Read the model definition and answer for the solid it produces. Units are mm, in the model's axes. A direction names the side the tool comes from. Round coordinates to 2 decimals unless told otherwise and drop trailing zeros. Loops run counter-clockwise (first coordinate to the right, second up) from the corner with the lowest first, then second, coordinate; pieces in that order, holes last. Notation, with made-up numbers: (41, 59) - (65, 59) arc R17 cw to (65, 80) - close; hole circle Ø9 at (-28, -0.75). An arc over 180 degrees is marked (long way). Use CSV: the item, a comma, the result in double quotes. Start each with the question number.
1. Determine the mould class of faces 4 (the flat face through (0, 1, 3.6)), 5 (the cylindrical face through (-3.67, -8.05, -0.02)), 6 (the conical face through (-3.412, 8.373, 2.942)), 7 (the flat face through (-3, 4.5, 0)) for opening direction Y: +Y half, -Y half, draft (parallel to the pull), parting line (faces both ways), or undercut.
2. Given pin 1 Ø1.2 at (x, z) = (2, -0.5) entering from +Y; pin 2 Ø1.7 at (x, z) = (-1.5, -0.5) entering from +Y; pin 3 Ø1.5 at (y, z) = (-3, 2.5) entering from +X, each flat-ended and moving along its own axis, determine where each tip first touches the part or whether it passes through.
3. Find section B-B (z = 0). State how many separate pieces and enclosed holes the cut face has, and give its area (3 significant figures).
4. Consider line 1 along Z through (x, y) = (1.25, -5.5); line 2 along X through (y, z) = (-6, 1); line 3 along X through (y, z) = (5.75, 2). Determine where each line is inside the solid, lowest interval first.
5. A tool of negligible diameter and unlimited length cuts with its end or side. For faces 1 (the flat face through (0, -1, -2.25)), 2 (the flat face through (-3, -4.5, 0)), 3 (the flat face through (-2.75, -5, 0)), from which of +Z, -Z, +X, -X, +Y, -Y can it reach the whole face along a straight path? Write none if from no direction.
6. Find section A-A (y = -0.5). Give the vertices of the cut face in (x, z), and give its area (3 significant figures).
7. Find section C-C (x = 0). Give the vertices of the cut face in (y, z) (3 decimals), and give its area (3 significant figures).
8. Find section D-D (y = 7.25). Give the vertices of the cut face in (x, z), and give its area (3 significant figures).
from build123d import *

# Parameters (mm, degrees)
SKETCH1_W                 = 8.2
SKETCH1_H                 = 7.2
BOSS_EXTRUDE1_DEPTH       = 8.5
SKETCH2_W                 = 0.25
SKETCH2_H                 = 0.25
SKETCH2_H_2               = 4
SKETCH2_W_2               = 5
CHAIN_DEPTH               = 15
F_2_5_MM_DOWEL_DEPTH      = 11.100495037
F_2_5_MM_DOWEL_DEPTH_BACK = 11.100495037
SKETCH3_R                 = 1.25
SKETCH4_R                 = 0.9
STEEL_CABLE_CHANNEL_DEPTH = 11.100495037
CRIMP_WINDOW_DEPTH        = 11.100495037
CRIMP_WINDOW_DEPTH_BACK   = 11.100495037
SKETCH7_W                 = 4.5
SKETCH7_H                 = 9
FILLET6_R                 = 0.75
FILLET7_R                 = 0.5
FILLET9_R                 = 0.5
FILLET3_R                 = 2
FILLET5_R                 = 1.5
CHAMFER1_SIZE             = 0.25
BOSS_EXTRUDE2_START       = 0.005
SKETCH5_R                 = 1.9
SKETCH5_R_2               = 0.9
BOSS_EXTRUDE2_DEPTH       = 0.005


with BuildPart() as part:
    # Sketch1 → Boss-Extrude1 (new, symmetric)
    with BuildSketch(Plane(origin=(0, 0, 0), x_dir=(1, 0, 0), z_dir=(0, 1, 0))):
        Rectangle(SKETCH1_W, SKETCH1_H)
    extrude(amount=BOSS_EXTRUDE1_DEPTH, both=True)

    # Sketch2 → chain (cut)
    with BuildSketch(Plane(origin=(0, 8.5, 0), x_dir=(1, 0, 0), z_dir=(0, 1, 0))):
        with Locations((-2.625, 2.125)):
            Rectangle(SKETCH2_W, SKETCH2_H)
        with Locations((-2.625, 0)):
            Rectangle(SKETCH2_W, SKETCH2_H_2)
        with Locations((0, 2.125)):
            Rectangle(SKETCH2_W_2, SKETCH2_H)
        Rectangle(SKETCH2_W_2, SKETCH2_H_2)
        with Locations((2.625, 2.125)):
            Rectangle(SKETCH2_W, SKETCH2_H)
        with Locations((2.625, 0)):
            Rectangle(SKETCH2_W, SKETCH2_H_2)
        with Locations((2.625, -2.125)):
            Rectangle(SKETCH2_W, SKETCH2_H)
        with Locations((0, -2.125)):
            Rectangle(SKETCH2_W_2, SKETCH2_H)
        with Locations((-2.625, -2.125)):
            Rectangle(SKETCH2_W, SKETCH2_H)
    extrude(amount=-CHAIN_DEPTH, mode=Mode.SUBTRACT)

    # Sketch3 → 2.5 mm dowel (cut, two sides: drawn at the far end of the back side and taken through both)
    with BuildSketch(Plane.XY.offset(-F_2_5_MM_DOWEL_DEPTH_BACK)):
        with Locations((0, 5)):
            Circle(SKETCH3_R)
    extrude(amount=F_2_5_MM_DOWEL_DEPTH + F_2_5_MM_DOWEL_DEPTH_BACK, mode=Mode.SUBTRACT)

    # Sketch4 → steel cable channel (cut, through all)
    with BuildSketch(Plane(origin=(0, 0, 0), x_dir=(1, 0, 0), z_dir=(0, 1, 0))):
        with Locations(Location((0, 0, 0), (0, 0, 270))):
            Circle(SKETCH4_R)
    extrude(amount=-STEEL_CABLE_CHANNEL_DEPTH, mode=Mode.SUBTRACT)

    # Sketch7 → crimp window (cut, two sides: drawn at the far end of the back side and taken through both)
    with BuildSketch(Plane.ZY.offset(-CRIMP_WINDOW_DEPTH_BACK)):
        Rectangle(SKETCH7_W, SKETCH7_H)
    extrude(amount=CRIMP_WINDOW_DEPTH + CRIMP_WINDOW_DEPTH_BACK, mode=Mode.SUBTRACT)

    # Fillet6
    fillet6_edges = [part.edges().sort_by_distance(p)[0] for p in [
        (-2.75, -5.5, -2.25),
        (2.75, -5.5, -2.25),
        (2.75, -5.5, 2.25),
        (-2.75, -5.5, 2.25),
        (-2.75, 6.5, -2.25),
        (-2.75, 6.5, 2.25),
        (2.75, 6.5, 2.25),
        (2.75, 6.5, -2.25),
    ]]
    fillet(fillet6_edges, radius=FILLET6_R)

    # Fillet7
    fillet7_edges = [part.edges().sort_by_distance(p)[0] for p in [
        (2.75, -6.5, 0),
        (2.530330086, -6.5, -2.030330086),
        (2.530330086, -6.5, 2.030330086),
        (-2.530330086, -6.5, 2.030330086),
        (-2.530330086, -6.5, -2.030330086),
        (0, -6.5, -2.25),
        (0, -6.5, 2.25),
        (-2.75, -6.5, 0),
    ]]
    fillet(fillet7_edges, radius=FILLET7_R)

    # Fillet9
    fillet9_edges = [part.edges().sort_by_distance(p)[0] for p in [
        (3.05, 4.5, -2.25),
        (3.05, -4.5, 2.25),
        (3.05, 4.5, 2.25),
        (-3.05, 4.5, 2.25),
        (3.05, -4.5, -2.25),
        (-3.05, -4.5, -2.25),
        (-3.05, 4.5, -2.25),
        (-3.05, -4.5, 2.25),
    ]]
    fillet(fillet9_edges, radius=FILLET9_R)

    # Fillet3
    # the kernel refuses this fillet: 2 mm, written as the material it takes off along each edge
    with BuildSketch(Plane(origin=(-4.1, 13.5, -3.6), x_dir=(1, 0, 0), z_dir=(0, -1, 0)), Plane(origin=(4.1, -13.5, -3.6), x_dir=(-1, 0, 0), z_dir=(0, 1, 0))) as fillet3_piece_1:
        with BuildLine():
            CenterArc((FILLET3_R, FILLET3_R), FILLET3_R, 180, 90)
            Line((0, FILLET3_R), (0, 0))
            Line((0, 0), (FILLET3_R, 0))
        make_face()
    extrude(amount=27, mode=Mode.SUBTRACT)
    with BuildSketch(Plane(origin=(-4.1, 13.5, 3.6), x_dir=(1, 0, 0), z_dir=(0, -1, 0)), Plane(origin=(4.1, -13.5, 3.6), x_dir=(-1, 0, 0), z_dir=(0, 1, 0))) as fillet3_piece_2:
        with BuildLine():
            CenterArc((FILLET3_R, -FILLET3_R), FILLET3_R, 90, 90)
            Line((0, -FILLET3_R), (0, 0))
            Line((0, 0), (FILLET3_R, 0))
        make_face()
    extrude(amount=27, mode=Mode.SUBTRACT)

    # Fillet5
    fillet5_edges = [part.edges().sort_by_distance(p)[0] for p in [
        (-4.1, -8.5, 0),
        (4.1, -8.5, 0),
        (0, -8.5, 3.6),
        (0, -8.5, -3.6),
        (3.514213562, -8.5, 3.014213562),
        (3.514213562, -8.5, -3.014213562),
        (-3.514213562, -8.5, 3.014213562),
        (-3.514213562, -8.5, -3.014213562),
    ]]
    fillet(fillet5_edges, radius=FILLET5_R)

    # Chamfer1
    chamfer1_edges = [part.edges().sort_by_distance(p)[0] for p in [
        (2.530330086, 8.5, -2.030330086),
        (-2.530330086, 8.5, -2.030330086),
        (2.530330086, 8.5, 2.030330086),
        (-2.530330086, 8.5, 2.030330086),
        (-4.1, 8.5, 0),
        (0, 8.5, -3.6),
        (4.1, 8.5, 0),
        (0, 8.5, 3.6),
        (3.514213562, 8.5, 3.014213562),
        (3.514213562, 8.5, -3.014213562),
        (-3.514213562, 8.5, 3.014213562),
        (-3.514213562, 8.5, -3.014213562),
        (0, 8.5, -2.25),
        (2.75, 8.5, 0),
        (-2.75, 8.5, 0),
        (0, 8.5, 2.25),
    ]]
    chamfer(chamfer1_edges, length=CHAMFER1_SIZE)

    # Sketch5 → Boss-Extrude2 (add)
    with BuildSketch(Plane(origin=(0, -6.5, 0), x_dir=(1, 0, 0), z_dir=(0, 1, 0)).offset(BOSS_EXTRUDE2_START)):
        Circle(SKETCH5_R)
        with Locations(Location((0, 0, 0), (0, 0, 270))):
            Circle(SKETCH5_R_2, mode=Mode.SUBTRACT)
    extrude(amount=-BOSS_EXTRUDE2_DEPTH)


solid = part.part
Filled sheet:
1,face 4,"draft"
1,face 5,"-Y half"
1,face 6,"+Y half"
1,face 7,"undercut"
2,pin 1,"stops at y = -6.36"
2,pin 2,"stops at y = -6.49"
2,pin 3,"stops at x = 3.99"
3,separate pieces,"4"
3,enclosed holes,"0"
3,area,"28.0 mm²"
4,line 1,"z = -3.6 to -2.25, 2.25 to 3.6"
4,line 2,"x = -4.1 to -2.75, 2.75 to 4.1"
4,line 3,"x = -4.06 to -2.56, 2.56 to 4.06"
5,face 1,"none"
5,face 2,"+X, -X"
5,face 3,"+Y"
6,outline,"(-3.99, -2.25) arc R2 ccw to (-2.1, -3.6) - (2.1, -3.6) arc R2 ccw to (3.99, -2.25) - close; (-3.99, 2.25) - (3.99, 2.25) arc R2 ccw to (2.1, 3.6) - (-2.1, 3.6) arc R2 ccw to start"
6,area,"18.8 mm²"
7,outline,"(-8.5, -2.1) arc R1.5 ccw to (-7, -3.6) - (3.75, -3.6) - (3.75, -2.25) - (-6, -2.25) arc R0.5 cw to (-6.495, -1.821) - (-6.495, -0.9) - (-8.5, -0.9) - close; (-8.5, 0.9) - (-6.495, 0.9) - (-6.495, 1.821) arc R0.5 cw to (-6, 2.25) - (3.75, 2.25) - (3.75, 3.6) - (-7, 3.6) arc R1.5 ccw to (-8.5, 2.1) - close; (6.25, -3.6) - (8.25, -3.6) - (8.5, -3.35) - (8.5, -2.5) - (8.25, -2.25) - (6.25, -2.25) - close; (6.25, 2.25) - (8.25, 2.25) - (8.5, 2.5) - (8.5, 3.35) - (8.25, 3.6) - (6.25, 3.6) - close"
7,area,"43.6 mm²"
8,outline,"(-4.1, -1.6) arc R2 ccw to (-2.1, -3.6) - (2.1, -3.6) arc R2 ccw to (4.1, -1.6) - (4.1, 1.6) arc R2 ccw to (2.1, 3.6) - (-2.1, 3.6) arc R2 ccw to (-4.1, 1.6) - close; hole (-2.75, -1.5) arc R0.75 ccw to (-2, -2.25) - (2, -2.25) arc R0.75 ccw to (2.75, -1.5) - (2.75, 1.5) arc R0.75 ccw to (2, 2.25) - (-2, 2.25) arc R0.75 ccw to (-2.75, 1.5) - close"
8,area,"31.3 mm²"
